Work out the finished part from the listing and answer in its coordinate system (mm). A direction names the side the tool comes from. Give positions to 0.01 mm unless a question says otherwise; leave off trailing zeros. Loops run counter-clockwise (first coordinate to the right, second up) from the corner with the lowest first, then second, coordinate; pieces in that order, holes last. Notation, with made-up numbers: M -12,-33.75 L -6,-33.75 A27 ccw -6,-8.75 Z; hole C 12.5,46 d10. An arc over 180 degrees is marked long. Answer in a Markdown table with one row per item. Add a question column.
from build123d import *

# Parameters (mm, degrees)
SKETCH2_R         = 3.207274827
HEX_DIE_DEPTH     = 4.3
FLANGEHEXFILLET_R = 0.2
SKETCH4_R         = 2.40625
INDENT_DEPTH      = 0.358333333


with BuildPart() as part:
    # BodySke → Base-Revolve (revolve)
    with BuildSketch(Plane.XY, mode=Mode.PRIVATE) as base_revolve_sk:
        Polygon((4.3, 2), (4.3, 3.17551963), (0.245673873, 3.17551963), (0, 2.75), (0, 0), (20.3, 0), (20.3, 2), align=None)
    revolve(base_revolve_sk.sketch.rotate(Axis((-25.4, 0, 0), (1, 0, 0)), 90), axis=Axis((-25.4, 0, 0), (1, 0, 0)))

    # Sketch2 → Hex-Die (cut)
    with BuildSketch(Plane(origin=(0, 0, 0), x_dir=(0, 0, -1), z_dir=(1, 0, 0))):
        Circle(SKETCH2_R)
        Polygon((-2.75, 1.587713247), (0, 3.175426494), (2.75, 1.587713247), (2.75, -1.587713247), (0, -3.175426494), (-2.75, -1.587713247), align=None, mode=Mode.SUBTRACT)
    extrude(amount=HEX_DIE_DEPTH, mode=Mode.SUBTRACT)

    # Sketch5 → Flange (revolve)
    with BuildSketch(Plane.XY, mode=Mode.PRIVATE) as flange_sk:
        with BuildLine():
            Line((2.243064243, 0), (3.718092214, 4.052606043))
            ThreePointArc((3.718092214, 4.052606043), (4.052094453, 4.245442326), (4.3, 3.95))
            Line((4.3, 3.95), (4.3, 0))
            Line((4.3, 0), (2.243064243, 0))
        make_face()
    revolve(flange_sk.sketch.rotate(Axis((0, 0, 0), (1, 0, 0)), 90), axis=Axis((0, 0, 0), (1, 0, 0)))

    # FlangeHexFillet
    flangehexfillet_edges = [part.edges().sort_by_distance(p)[0] for p in [
        (3.285203168, 0.797319684, 2.75),
        (3.24398239, 2.381569871, 1.375),
        (3.24398239, 2.381569871, -1.375),
        (3.243982387, 0, -2.75),
        (3.24398239, -2.381569871, -1.375),
        (3.24398239, -2.381569871, 1.375),
        (3.285203168, -0.797319684, 2.75),
    ]]
    fillet(flangehexfillet_edges, radius=FLANGEHEXFILLET_R)

    # Sketch4 → Indent (cut)
    with BuildSketch(Plane(origin=(0, 0, 0), x_dir=(0, 0, -1), z_dir=(1, 0, 0))):
        with Locations(Location((0, 0, 0), (0, 0, 180))):
            Circle(SKETCH4_R)
    extrude(amount=INDENT_DEPTH, mode=Mode.SUBTRACT)


solid = part.part
(1) Consider line 1 along X through (y, z) = (-2.25, -1); line 2 along X through (y, z) = (0, -0.25); line 3 along Y through (x, z) = (0.2, 0). Determine where each line is inside the solid, lowest interval first. Write a range as from..to.
(2) The mould has two halves that part along Z. Classify faces 5 (the face through (0.358, 0, 0)), 6 (the face through (1.602, -2.37, -1.394)), 7 (the face through (0.177, 1.464, -1.91)), 8 (the face through (20.3, 0, 0)): pulls with the +Z half, pulls with the -Z half, needs draft (parallel to the pull), parting line crosses it, or undercut.
(3) Section A-A, the plane x = 2.5 is taken. Determine the outline of the cut face in (y, z).
(4) Each of these flat-tipped pins is pushed along its axis until it touches: P1, Ø1.6, axis at x = 1, y = 0.5, coming from the +Z side; P2, Ø5, axis at x = 14.5, z = 1.5, coming from the -Y side; P3, Ø1.6, axis at x = 1.5, y = -0.5, coming from the -Z side; P4, Ø1, axis at x = 16.5, z = -3, coming from the +Y side. Where does it stop, or does it pass through?
(5) Which of the six approach directions +Z, -Z, +X, -X, +Y, -Y give full straight-line access (tool end or side, diameter ignored) to faces 1 (the face through (1.602, 2.37, 1.394)), 2 (the face through (1.6, -2.39, 1.36)), 3 (the face through (1.6, 2.39, -1.36)), 4 (the face through (12, 2, 0))?
(6) Section B-B, the plane x = 5 is taken. Determine the outline of the cut face in (y, z).
Numbers:
| question | item | result |
|---|---|---|
| 1 | line 1 | x = 0..4.3 |
| 1 | line 2 | x = 0.36..20.3 |
| 1 | line 3 | y = -3.1..-2.41, 2.41..3.1 |
| 2 | face 5 | undercut |
| 2 | face 6 | pulls with the -Z half |
| 2 | face 7 | undercut |
| 2 | face 8 | needs draft |
| 3 | outline | M -3.18,0 L -1.59,-2.75 L 1.59,-2.75 L 3.18,0 L 1.59,2.75 L -1.59,2.75 Z |
| 4 | P1 | stops at z = 2.75 |
| 4 | P2 | stops at y = -2 |
| 4 | P3 | stops at z = -2.75 |
| 4 | P4 | passes through |
| 5 | face 1 | +Z, -X, +Y |
| 5 | face 2 | +Z, -X, -Y |
| 5 | face 3 | -Z, -X, +Y |
| 5 | face 4 | +X |
| 6 | outline | C 0,0 d4 |
